For this review, take the finished solid that the model builds, in its own axes (mm). A direction names the side the tool comes from. Give positions to 0.01 mm unless a question says otherwise; leave off trailing zeros. Write each loop counter-clockwise with the first axis right and the second up, starting at its lowest first coordinate (ties: lowest second). Pieces come first, ordered by that corner, then holes.
Autodesk Inventor part; units mm, degrees
ref_plane "YZ Plane" through (0, 0, 0) normal (1, 0, 0) x (0, 1, 0)
ref_plane "XZ Plane" through (0, 0, 0) normal (0, 1, 0) x (-1, 0, 0)
ref_plane "XY Plane" through (0, 0, 0) normal (0, 0, 1) x (1, 0, 0)
sketch "Sketch1" plane through (0, 0, 0) normal (0, 1, 0) x (-1, 0, 0)
  circle A0 centre (0, 0) radius 7.5
  dimension "d0" = 15
extrude "Extrusion1" add sketch "Sketch1" along normal blind 3
sketch "Sketch2" plane through (0, 0, 0) normal (0, -1, 0) x (1, 0, 0)
  circle A0 centre (0, 0) radius 7.5
  circle A1 centre (0, 0) radius 2.3
  dimension "d3" = 4.6
extrude "Extrusion2" add sketch "Sketch2" along normal blind 3.6 contours A1
sketch "Sketch3" plane through (0, -3.6, 0) normal (0, -1, 0) x (1, 0, 0)
  circle A0 centre (0, 0) radius 2.3
  line L0 (-2.3, 4.6637) -> (-2.3, -5.1059)
  line L1 (2.3, 4.6637) -> (2.3, -5.1059)
  line L2 (0, 15.7328) -> (0, -15.032) construction
  circle A1 centre (0, 0) radius 7.5 construction
  arc A2 (-3, 6.8739) -> (-3, -6.8739) centre (0, 0) ccw construction
  arc A3 (3, -6.8739) -> (3, 6.8739) centre (0, 0) ccw construction
  arc A4 (2.3, 4.6637) -> (-2.3, 4.6637) centre (0, 0) ccw
  arc A5 (-2.3, -5.1059) -> (2.3, -5.1059) centre (0, 0) ccw
  dimension "d13" = 5.2
  dimension "d19" = 5.6
extrude "Extrusion3" add sketch "Sketch3" along normal blind 2.8
fillet "Fillet2" radius 1.2 4 edges at (-2.3, -5, 4.6637) (2.3, -5, 4.6637) (-2.3, -5, -5.1059) (2.3, -5, -5.1059)
equation "\"d0\" = HeadConnectorOuterSize"
equation "\"d1\" = EarConnectorHeight"
equation "\"d3\" = HeadConnectorWidth - HeadConnectorTolerance"
equation "\"d4\" = HeadConnectorOuterHeight + 3 * HeadConnectorTolerance"
equation "\"d13\" = 0.5 * HeadConnectorDiam - 4 * HeadConnectorTolerance"
equation "\"d19\" = 0.5 * HeadConnectorDiam - 2 * HeadConnectorTolerance"
equation "\"d10\" = HeadConnectorHeight - HeadConnectorTolerance"
equation "\"d20\" = 0.2 * HeadConnectorProportion"
equation "\"EarConnectorHeight\" = 0.5 * HeadConnectorProportion"
properties part number "EarConnector"
(1) We need section D-D (y = -1.5). Write out the cut boundary in (x, z).
(2) Tool access review of faces 4 (the cylindrical face through (-2.055, -5.02, -4.986)), 5 (the cylindrical face through (0, -5, -5.6)), 6 (the cylindrical face through (2.065, -5.02, 4.56)): name each direction out of +Z, -Z, +X, -X, +Y, -Y from which nothing blocks a thin tool from reaching the whole face with its end or side.
(3) The part is to be moulded in two halves that separate along Y. For faces 1 (the cylindrical face through (-1.825, -1.775, 1.4)), 2 (the flat face through (0, 3, 0)), 3 (the cylindrical face through (-2.05, -5.02, 4.58)), say which applies: +Y half, -Y half, draft (parallel to the pull), parting line (faces both ways), or undercut.
(4) Clearance check with flat-ended pins moving along their axes: pin 1 Ø0.8 at (y, z) = (-4.5, 0) entering from +X; pin 2 Ø3 at (y, z) = (-5.5, 0.5) entering from -X; pin 3 Ø5 at (x, y) = (2.5, 1) entering from -Z; pin 4 Ø3 at (x, y) = (1.5, -4) entering from -Z. State where each tip first meets the part, or that it passes through.
(5) We need section B-B (y = -4.5). Write out the cut boundary in (x, z).
(6) We need section A-A (x = 0). Write out the cut boundary in (y, z), and give its area (3 significant figures).
(7) For L1, parallel to Y at x = -2.25, z = -1.5; L2, parallel to Y at x = -4.5, z = -4.75; L3, parallel to X at y = -5, z = 2.75, list the stretches that pass through material, from the lowest coordinate up.
(8) We need section C-C (z = -1). Write out the cut boundary in (x, y), and give its area (3 significant figures).
The answers:
1. outline: circle Ø4.6 at (0, 0)
2. face 4: -Z, -X, -Y
2. face 5: -Z, -Y
2. face 6: +Z, +X, -Y
3. face 1: undercut
3. face 2: +Y half
3. face 3: draft
4. pin 1: stops at x = 2.3
4. pin 2: stops at x = -2.3
4. pin 3: stops at z = -7.5
4. pin 4: stops at z = -5.6
5. outline: (-2.3, -4.26) arc R1.2 ccw to (-1.4, -5.42) arc R5.6 ccw to (1.4, -5.42) arc R1.2 ccw to (2.3, -4.26) - (2.3, 3.85) arc R1.2 ccw to (1.43, 5) arc R5.2 ccw to (-1.43, 5) arc R1.2 ccw to (-2.3, 3.85) - close
6. outline: (-6.4, -5.6) - (-3.6, -5.6) - (-3.6, -2.3) - (0, -2.3) - (0, -7.5) - (3, -7.5) - (3, 7.5) - (0, 7.5) - (0, 2.3) - (-3.6, 2.3) - (-3.6, 5.2) - (-6.4, 5.2) - close
6. area: 91.8 mm2
7. L1: y = -6.4 to -3.6, 0 to 3
7. L2: y = 0 to 3
7. L3: x = -2.3 to 2.3
8. outline: (-7.43, 0) - (-2.07, 0) - (-2.07, -3.6) - (-2.3, -3.6) - (-2.3, -6.4) - (2.3, -6.4) - (2.3, -3.6) - (2.07, -3.6) - (2.07, 0) - (7.43, 0) - (7.43, 3) - (-7.43, 3) - close
8. area: 72.4 mm2
